The listing builds one solid part. Answer for the finished solid, in the listing's coordinates (mm). A direction names the side the tool comes from. Coordinates: 2 decimals unless noted, no trailing zeros. Loops run counter-clockwise (first coordinate to the right, second up) from the corner with the lowest first, then second, coordinate; pieces in that order, holes last. Notation, with made-up numbers: (35, -27.5) -> (90, -27.5) arc R28 cw to (90, 5.5) -> close; hole circle Ø11 at (44, -4.75). An arc over 180 degrees is marked (long way). Answer in a Markdown table with one row per item.
```python
from build123d import *

# Parameters (mm, degrees)
SKETCH_1_R          = 21
EXTRUDE_1_DEPTH     = 17.5
SKETCH_2_W          = 1
SKETCH_2_H          = 31
SKETCH_3_R          = 12
CUT_EXTRUDE_1_DEPTH = 10
SKETCH_15_R         = 10
CUT_EXTRUDE_3_DEPTH = 39.820097888
SCALE1_SCALE        = 2


with BuildPart() as part:
    # 草图1 → 凸台-拉伸1 (new, symmetric)
    with BuildSketch(Plane(origin=(0, 0, 0), x_dir=(1, 0, 0), z_dir=(0, 1, 0))):
        with Locations(Location((0, 0, 0), (0, 0, 270))):
            Circle(SKETCH_1_R)
    extrude(amount=EXTRUDE_1_DEPTH, both=True)

    # 草图2 → 切除-旋转1 (revolve, cut)
    with BuildSketch(Plane.XY, mode=Mode.PRIVATE) as cut_revolve_1_sk:
        with Locations((20.5, 0)):
            Rectangle(SKETCH_2_W, SKETCH_2_H)
    revolve(cut_revolve_1_sk.sketch.rotate(Axis((0, 17.5, 0), (0, -1, 0)), 90), axis=Axis((0, 17.5, 0), (0, -1, 0)), mode=Mode.SUBTRACT)

    # 草图3 → 切除-拉伸1 (cut)
    with BuildSketch(Plane(origin=(0, 17.5, 0), x_dir=(1, 0, 0), z_dir=(0, 1, 0))):
        with Locations(Location((0, 0, 0), (0, 0, 270))):
            Circle(SKETCH_3_R)
    cut_extrude_1 = extrude(amount=-CUT_EXTRUDE_1_DEPTH, mode=Mode.SUBTRACT)

    # 草图15 → 切除-拉伸3 (cut, through all)
    with BuildSketch(Plane(origin=(0, 7.5, 0), x_dir=(1, 0, 0), z_dir=(0, 1, 0))):
        with Locations(Location((0, 0, 0), (0, 0, 270))):
            Circle(SKETCH_15_R)
    extrude(amount=-CUT_EXTRUDE_3_DEPTH, mode=Mode.SUBTRACT)

    # 镜向1: 切除-拉伸1 across plane
    add(cut_extrude_1.mirror(Plane.ZX), mode=Mode.SUBTRACT)


with BuildPart() as part_1:
    # Scale1: scaled about (0, 0, 0)
    add(part.part.scale(SCALE1_SCALE))


solid = part_1.part
```
Item 1: A tool of negligible diameter and unlimited length cuts with its end or side. For faces 1 (the face through (7.21, -25.14, 22.89)), 2 (the face through (7.21, 25.14, 22.89)), 3 (the face through (15.4, 31, -37.1)), from which of +Z, -Z, +X, -X, +Y, -Y can it reach the whole face along a straight path? Write none if from no direction.
Findings below:
| item | result |
|---|---|
| face 1 | -Y |
| face 2 | +Y |
| face 3 | none |
Item 2: A cutting plane is placed at C-C, the plane y = -29. Determine the outline of the cut face in (x, z), plus the area to 3 significant figures.
Findings below:
| item | result |
|---|---|
| outline | circle Ø80 at (0, 0); hole circle Ø48 at (0, 0) |
| area | 3,220 mm2 |
Item 3: Flat-ended cylindrical pins translate along their axes: pin 1 Ø24 at (x, z) = (0, 0) entering from -Y; pin 2 Ø4 at (x, y) = (23.5, -16.5) entering from +Z; pin 3 Ø12 at (x, y) = (-1.5, 17) entering from -Z; pin 4 Ø12 at (y, z) = (-14.5, 19.5) entering from +X. Find the tip coordinate at first contact, or state that the pin passes through.
Findings below:
| item | result |
|---|---|
| pin 1 | passes through |
| pin 2 | stops at z = 33.73 |
| pin 3 | stops at z = -40 |
| pin 4 | stops at x = 37.65 |
Item 4: A cutting plane is placed at B-B, the plane z = 0. Determine the outline of the cut face in (x, y).
Findings below:
| item | result |
|---|---|
| outline | (-42, -35) -> (-24, -35) -> (-24, -15) -> (-20, -15) -> (-20, 15) -> (-24, 15) -> (-24, 35) -> (-42, 35) -> (-42, 31) -> (-40, 31) -> (-40, -31) -> (-42, -31) -> close; (20, -15) -> (24, -15) -> (24, -35) -> (42, -35) -> (42, -31) -> (40, -31) -> (40, 31) -> (42, 31) -> (42, 35) -> (24, 35) -> (24, 15) -> (20, 15) -> close |
Item 5: A cutting plane is placed at D-D, the plane y = 1. Determine the outline of the cut face in (x, z), plus the area to 3 significant figures.
Findings below:
| item | result |
|---|---|
| outline | circle Ø80 at (0, 0); hole circle Ø40 at (0, 0) |
| area | 3,770 mm2 |
Item 6: A cutting plane is placed at A-A, the plane x = 0. Determine the outline of the cut face in (y, z).
Findings below:
| item | result |
|---|---|
| outline | (-35, -42) -> (-31, -42) -> (-31, -40) -> (31, -40) -> (31, -42) -> (35, -42) -> (35, -24) -> (15, -24) -> (15, -20) -> (-15, -20) -> (-15, -24) -> (-35, -24) -> close; (-35, 24) -> (-15, 24) -> (-15, 20) -> (15, 20) -> (15, 24) -> (35, 24) -> (35, 42) -> (31, 42) -> (31, 40) -> (-31, 40) -> (-31, 42) -> (-35, 42) -> close |
Item 7: Determine the mould class of faces 4 (the face through (12.62, -32.97, 40.06)), 5 (the face through (15.4, -31, -37.1)), 6 (the face through (20, -15, -5)) for opening direction X: +X half, -X half, draft (parallel to the pull), parting line (faces both ways), or undercut.
Findings below:
| item | result |
|---|---|
| face 4 | parting line |
| face 5 | draft |
| face 6 | undercut |
Item 8: Find the intervals of material crossed by probe 1 along X at (y, z) = (-26.25, 0); probe 2 along Y at (x, z) = (-16.5, 38.5); probe 3 along X at (y, z) = (5.75, 0), in increasing order.
Findings below:
| item | result |
|---|---|
| probe 1 | x = -40 to -24, 24 to 40 |
| probe 2 | y = -35 to -31, 31 to 35 |
| probe 3 | x = -40 to -20, 20 to 40 |
